from build123d import *

# Parameters (mm, degrees)
SKETCH1_W           = 101.6
SKETCH1_H           = 76.2
BOSS_EXTRUDE1_DEPTH = 38.1
SKETCH3_W           = 97.6
SKETCH3_H           = 72.2
CUT_EXTRUDE1_DEPTH  = 75.053089065
SKETCH7_R           = 2.54
CUT_EXTRUDE2_DEPTH  = 2
SKETCH9_R           = 4
CUT_EXTRUDE3_DEPTH  = 2
SKETCH11_R          = 3.175
CUT_EXTRUDE4_DEPTH  = 2
FILLET1_R           = 5
FILLET2_R           = 5


with BuildPart() as part:
    # Sketch1 → Boss-Extrude1 (new body)
    with BuildSketch(Plane(origin=(0, 0, 0), x_dir=(1, 0, 0), z_dir=(0, 1, 0))):
        Rectangle(SKETCH1_W, SKETCH1_H)
    extrude(amount=BOSS_EXTRUDE1_DEPTH)

    # Sketch3 → Cut-Extrude1 (cut, through all)
    with BuildSketch(Plane(origin=(0, 38.1, 0), x_dir=(1, 0, 0), z_dir=(0, 1, 0))):
        Rectangle(SKETCH3_W, SKETCH3_H)
    extrude(amount=-CUT_EXTRUDE1_DEPTH, mode=Mode.SUBTRACT)

    # Sketch7 → Cut-Extrude2 (cut)
    with BuildSketch(Plane(origin=(50.8, 0, 0), x_dir=(0, 0, -1), z_dir=(1, 0, 0))):
        with Locations((-8.255, 19.05)):
            Circle(SKETCH7_R)
        with Locations((8.255, 19.05)):
            Circle(SKETCH7_R)
    extrude(amount=-CUT_EXTRUDE2_DEPTH, mode=Mode.SUBTRACT)

    # Sketch9 → Cut-Extrude3 (cut)
    with BuildSketch(Plane.ZY.offset(50.8)):
        with Locations((0, 19.05)):
            Circle(SKETCH9_R)
    extrude(amount=-CUT_EXTRUDE3_DEPTH, mode=Mode.SUBTRACT)

    # Sketch11 → Cut-Extrude4 (cut)
    with BuildSketch(Plane.XY.offset(38.1)):
        with Locations((-29.061160139, 19.05)):
            Circle(SKETCH11_R)
    extrude(amount=-CUT_EXTRUDE4_DEPTH, mode=Mode.SUBTRACT)

    # Fillet1
    fillet1_edges = [part.edges().sort_by_distance(p)[0] for p in [
        (50.8, 19.05, 38.1),
        (-50.8, 19.05, 38.1),
        (-50.8, 19.05, -38.1),
        (50.8, 19.05, -38.1),
    ]]
    fillet(fillet1_edges, radius=FILLET1_R)

    # Fillet2
    fillet2_edges = [part.edges().sort_by_distance(p)[0] for p in [
        (48.8, 19.05, 36.1),
        (-48.8, 19.05, 36.1),
        (-48.8, 19.05, -36.1),
        (48.8, 19.05, -36.1),
    ]]
    fillet(fillet2_edges, radius=FILLET2_R)


solid = part.part
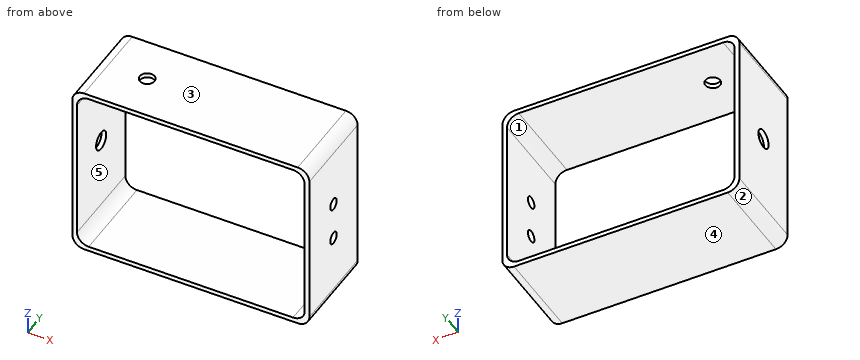
Verification items for the finished model (mm, model axes). Face numbers are marked on the shaded views. A direction names the side the tool comes from. Coordinates: 2 decimals unless noted, no trailing zeros. Loops run counter-clockwise (first coordinate to the right, second up) from the corner with the lowest first, then second, coordinate; pieces in that order, holes last. Notation, with made-up numbers: M 54,50.25 L 82,50.25 A5 ccw 82,58.25 Z; hole C 61.25,89 d9. An arc over 180 degrees is marked long. One line per item, written item: value.
1. Gauge pin test, flat end, axial feed: P1, Ø4.5, axis at y = 19.05, z = -8.255, coming from the +X side. Record the tip position at first contact, or that the pin passes through.
Answers follow:
P1: x = -48.8
2. Section check A-A on z = -30. Record the cut outline in (x, y).
Answers follow:
outline: M -50.8,0 L -48.8,0 L -48.8,38.1 L -50.8,38.1 Z; M 48.8,0 L 50.8,0 L 50.8,38.1 L 48.8,38.1 Z
3. Section check C-C on y = 19.05. Give the number of separate pieces and of enclosed holes in the cut face, plus the area to 3 significant figures.
Answers follow:
separate pieces: 4
enclosed holes: 0
area: 646 mm^2
4. Mould release check, pull along Z, two halves, no side actions. Record for the marked faces 3, 4 and 5: pulls with the +Z half, pulls with the -Z half, needs draft (parallel to the pull), parting line crosses it, or undercut.
Answers follow:
face 3: pulls with the +Z half
face 4: pulls with the -Z half
face 5: undercut
5. Section check B-B on x = 34.5. Record the cut outline in (y, z).
Answers follow:
outline: M 0,-38.1 L 38.1,-38.1 L 38.1,-36.1 L 0,-36.1 Z; M 0,36.1 L 38.1,36.1 L 38.1,38.1 L 0,38.1 Z
6. Material ranges on line 1 along Z through (x, y) = (-22.5, 11); line 2 along X through (y, z) = (7, -22.5); line 3 along Z through (x, y) = (-49, 19), recorded low to high. Write a range as from..to.
Answers follow:
line 1: -38.1..-36.1, 36.1..38.1
line 2: -50.8..-48.8, 48.8..50.8
line 3: -36.94..-4, 4..36.94
7. Set-up check for the marked faces 1 and 2: record each of +Z, -Z, +X, -X, +Y, -Y from which the full face is reachable in a straight line by a thin tool's end or side.
Answers follow:
face 1: +Y, -Y
face 2: -Z, -X, +Y, -Y
8. Section check D-D on z = 0. Record the cut outline in (x, y), plus the area to 3 significant figures.
Answers follow:
outline: M -50.8,0 L -48.8,0 L -48.8,15.05 L -50.8,15.05 Z; M -50.8,23.05 L -48.8,23.05 L -48.8,38.1 L -50.8,38.1 Z; M 48.8,0 L 50.8,0 L 50.8,38.1 L 48.8,38.1 Z
area: 136 mm^2
